```python
from build123d import *

# Parameters (mm, degrees)
SKETCH085_R     = 10
SKETCH085_R_2   = 1.6
SKETCH085_R_3   = 2.2
SKETCH085_R_4   = 2.5
PAD046_DEPTH    = 6.6
POCKET005_DEPTH = 2
CHAMFER002_SIZE = 0.2
CHAMFER003_SIZE = 0.4
CHAMFER004_SIZE = 0.2


with BuildPart() as part:
    # Sketch085 → Pad046 (new body)
    with BuildSketch(Plane.XY):
        Circle(SKETCH085_R)
        with Locations((0, 7)):
            Circle(SKETCH085_R_2, mode=Mode.SUBTRACT)
        with Locations((7, 0)):
            Circle(SKETCH085_R_3, mode=Mode.SUBTRACT)
        with Locations((0, -7)):
            Circle(SKETCH085_R_2, mode=Mode.SUBTRACT)
        with Locations((-7, 0)):
            Circle(SKETCH085_R_3, mode=Mode.SUBTRACT)
        Circle(SKETCH085_R_4, mode=Mode.SUBTRACT)
    extrude(amount=-PAD046_DEPTH)

    # Sketch086 → Pocket005 (cut)
    with BuildSketch(Plane.XY):
        with BuildLine():
            ThreePointArc((-3, 7), (0, 4), (3, 7))
            Line((3, 7), (3, 10))
            ThreePointArc((3, 10), (0, 13), (-3, 10))
            Line((-3, 10), (-3, 7))
        make_face()
        with BuildLine():
            ThreePointArc((3, -7), (0, -4), (-3, -7))
            Line((-3, -7), (-3, -10))
            ThreePointArc((-3, -10), (0, -13), (3, -10))
            Line((3, -10), (3, -7))
        make_face()
    extrude(amount=-POCKET005_DEPTH, mode=Mode.SUBTRACT)

    # Chamfer002
    chamfer002_edges = [part.edges().sort_by_distance(p)[0] for p in [
        (-1.6, 7, -2),
        (-1.6, -7, -2),
    ]]
    chamfer(chamfer002_edges, length=CHAMFER002_SIZE)

    # Chamfer003
    chamfer003_edges = [part.edges().sort_by_distance(p)[0] for p in [
        (4.8, 0, 0),
        (-9.2, 0, 0),
        (-2.5, 0, 0),
        (-1.6, 7, -6.6),
        (-2.5, 0, -6.6),
        (4.8, 0, -6.6),
        (-1.6, -7, -6.6),
        (-9.2, 0, -6.6),
    ]]
    chamfer(chamfer003_edges, length=CHAMFER003_SIZE)

    # Chamfer004
    chamfer004_edges = [part.edges().sort_by_distance(p)[0] for p in [
        (-10, 0, -6.6),
    ]]
    chamfer(chamfer004_edges, length=CHAMFER004_SIZE)


solid = part.part
```
Verification items for the finished model (mm, model axes). A direction names the side the tool comes from. Coordinates: 2 decimals unless noted, no trailing zeros. Loops run counter-clockwise (first coordinate to the right, second up) from the corner with the lowest first, then second, coordinate; pieces in that order, holes last. Notation, with made-up numbers: (80, 47.25) -> (129, 47.25) arc R26 ccw to (129, 67.25) -> close; hole circle Ø5 at (2.25, 53). An arc over 180 degrees is marked (long way). Answer in a Markdown table with one row per item. Add a question column.
1. Depth check by flat-ended pin: P1, Ø5, axis at x = 7, y = 0, coming from the +Z side; P2, Ø4, axis at x = 0, y = -7, coming from the +Z side; P3, Ø1.6, axis at y = -8, z = -0.5, coming from the -X side. Enter the tip coordinate at first touch or a pass-through.
2. Section check A-A, the plane x = 0. Give the number of separate pieces and of enclosed holes in the cut face, then the cut area to 3 significant figures.
3. Access from +Z, -Z, +X, -X, +Y, -Y to the whole of each face (thin tool, end or side, straight path). Record for faces 1 (the face through (-3, -8, -1)), 2 (the face through (-4.9, 0.66, -3.26)), 3 (the face through (-3, 8, -1)).
4. Section check C-C, the plane z = -3.5. Enter the section's corners in (x, y), then the cut area to 3 significant figures.
5. Material ranges on probe 1 along Y at (x, z) = (0, -3.85); probe 2 along X at (y, z) = (-1, -5.5); probe 3 along Z at (x, y) = (1.75, 5), recorded low to high. Write a range as [from, to].
6. Section check B-B, the plane z = -1.5. Enter the section's corners in (x, y).
7. Draft check along X on faces 4 (the face through (9.032, -0.843, -3.259)), 5 (the face through (-2.31, -2.04, -6.6)). Enter one of: +X half, -X half, draft (parallel to the pull), parting line (faces both ways), or undercut.
Derived:
| question | item | result |
|---|---|---|
| 1 | P1 | stops at z = -0.1 |
| 1 | P2 | stops at z = -2 |
| 1 | P3 | stops at x = -6.94 |
| 2 | separate pieces | 4 |
| 2 | enclosed holes | 0 |
| 2 | area | 44.8 mm² |
| 3 | face 1 | +Z, -Y |
| 3 | face 2 | +Z, -Z |
| 3 | face 3 | +Z, +Y |
| 4 | outline | circle Ø20 at (0, 0); hole circle Ø4.4 at (-7, 0); hole circle Ø5 at (0, 0); hole circle Ø3.2 at (0, -7); hole circle Ø3.2 at (0, 7); hole circle Ø4.4 at (7, 0) |
| 4 | area | 248 mm² |
| 5 | probe 1 | y = [-10, -8.6], [-5.4, -2.5], [2.5, 5.4], [8.6, 10] |
| 5 | probe 2 | x = [-9.95, -8.96], [-5.04, -2.29], [2.29, 5.04], [8.96, 9.95] |
| 5 | probe 3 | z = [-6.6, -2] |
| 6 | outline | (-3, -9.54) -> (-3, -7) arc R3 cw to (3, -7) -> (3, -9.54) arc R10 ccw to (3, 9.54) -> (3, 7) arc R3 cw to (-3, 7) -> (-3, 9.54) arc R10 ccw to start; hole circle Ø4.4 at (-7, 0); hole circle Ø5 at (0, 0); hole circle Ø4.4 at (7, 0) |
| 7 | face 4 | undercut |
| 7 | face 5 | draft |
